```python
from build123d import *

# Parameters (mm, degrees)
F0_W      = 100
F0_H      = 100
F1_DEPTH  = 10
F2_R      = 3.75
F3_DEPTH  = 5
F4_R      = 3.75
F5_DEPTH  = 5
F7_R      = 3.75
F8_DEPTH  = 5
F9_R      = 3.75
F10_DEPTH = 5
F11_R     = 3.75
F12_DEPTH = 5
F13_R     = 3.75
F14_DEPTH = 5
F6_R      = 3.75
F15_DEPTH = 5


with BuildPart() as f1:
    # F0 (on Front) → F1 (new body)
    with BuildSketch(Plane.XZ):
        Rectangle(F0_W, F0_H)
    extrude(amount=F1_DEPTH)

    # F2 (on face) → F3 (join)
    with BuildSketch(Plane.XZ.offset(10)):
        Circle(F2_R)
    extrude(amount=F3_DEPTH)

    # F4 (on face) → F5 (join)
    with BuildSketch(Plane.XZ.offset(10)):
        with Locations((18, 0)):
            Circle(F4_R)
    extrude(amount=F5_DEPTH)

    # F7 (on face) → F8 (join)
    with BuildSketch(Plane.XZ.offset(10)):
        with Locations((-4, -20)):
            Circle(F7_R)
    extrude(amount=F8_DEPTH)

    # F9 (on face) → F10 (join)
    with BuildSketch(Plane.XZ.offset(10)):
        with Locations((-28, -20)):
            Circle(F9_R)
    extrude(amount=F10_DEPTH)

    # F11 (on face) → F12 (join)
    with BuildSketch(Plane.XZ.offset(10)):
        with Locations((-28, 6)):
            Circle(F11_R)
    extrude(amount=F12_DEPTH)

    # F13 (on face) → F14 (join)
    with BuildSketch(Plane.XZ.offset(10)):
        with Locations((-28, 34)):
            Circle(F13_R)
    extrude(amount=F14_DEPTH)

    # F6 (on face) → F15 (join)
    with BuildSketch(Plane.XZ.offset(10)):
        with Locations((18, -20)):
            Circle(F6_R)
    extrude(amount=F15_DEPTH)


solid = f1.part
```
The listing builds one solid part. Answer for the finished solid, in the listing's coordinates (mm). A direction names the side the tool comes from. Give positions to 0.01 mm unless a question says otherwise; leave off trailing zeros. Order: outer loops, then holes, each group sorted by start corner. A loop starts at its lowest first (then second) coordinate and runs counter-clockwise, first axis right, second up. Notation, with made-up numbers: (14, 51) - (46, 51) arc R26 ccw to (46, 66) - close; hole circle Ø8 at (61, -11.75). An arc over 180 degrees is marked (long way). Answer in a Markdown table with one row per item. Add a question column.
Q1. The part is cut by section C-C (z = -20). Determine the outline of the cut face in (x, y).
Q2. For a pull along Z with two mould halves and no side action, classify faces 3 (the flat face through (-4, -15, -20)), 4 (the cylindrical face through (-28.81, -12.46, 30.34)), 5 (the flat face through (-1, -5, 50)) as released by +Z, released by -Z, zero draft, split by the parting line, or undercut.
Q3. Find the intervals of material crossed by line 1 along Y through (x, z) = (39, -6); line 2 along Z through (x, y) = (-1, -14.25), in increasing order. Write a range as [from, to].
Q4. Which of the six approach directions +Z, -Z, +X, -X, +Y, -Y give full straight-line access (tool end or side, diameter ignored) to faces 1 (the flat face through (18, -15, -20)), 2 (the cylindrical face through (-3.746, -12.465, 0.165))?
Q5. The part is cut by section D-D (x = 18). Determine the outline of the cut face in (y, z), then the cut area to 4 significant figures.
Q6. The part is cut by section A-A (z = 6). Determine the outline of the cut face in (x, y), then the cut area to 3 significant figures.
Q7. Given P1, Ø5, axis at x = -28.5, y = -13, coming from the -Z side, flat-ended and moving along its own axis, determine where the tip first touches the part or whether it passes through.
Q8. The part is cut by section B-B (x = -28). Determine the outline of the cut face in (y, z), then the cut area to 3 significant figures.
Determined:
| question | item | result |
|---|---|---|
| 1 | outline | (-50, -10) - (-31.75, -10) - (-31.75, -15) - (-24.25, -15) - (-24.25, -10) - (-7.75, -10) - (-7.75, -15) - (-0.25, -15) - (-0.25, -10) - (14.25, -10) - (14.25, -15) - (21.75, -15) - (21.75, -10) - (50, -10) - (50, 0) - (-50, 0) - close |
| 2 | face 3 | zero draft |
| 2 | face 4 | undercut |
| 2 | face 5 | released by +Z |
| 3 | line 1 | y = [-10, 0] |
| 3 | line 2 | z = [-22.25, -17.75], [-3.61, 3.61] |
| 4 | face 1 | +Z, -Z, +X, -X, -Y |
| 4 | face 2 | -Y |
| 5 | outline | (-15, -23.75) - (-10, -23.75) - (-10, -50) - (0, -50) - (0, 50) - (-10, 50) - (-10, 3.75) - (-15, 3.75) - (-15, -3.75) - (-10, -3.75) - (-10, -16.25) - (-15, -16.25) - close |
| 5 | area | 1,075 mm² |
| 6 | outline | (-50, -10) - (-31.75, -10) - (-31.75, -15) - (-24.25, -15) - (-24.25, -10) - (50, -10) - (50, 0) - (-50, 0) - close |
| 6 | area | 1,040 mm² |
| 7 | P1 | stops at z = -23.75 |
| 8 | outline | (-15, -23.75) - (-10, -23.75) - (-10, -50) - (0, -50) - (0, 50) - (-10, 50) - (-10, 37.75) - (-15, 37.75) - (-15, 30.25) - (-10, 30.25) - (-10, 9.75) - (-15, 9.75) - (-15, 2.25) - (-10, 2.25) - (-10, -16.25) - (-15, -16.25) - close |
| 8 | area | 1,110 mm² |
